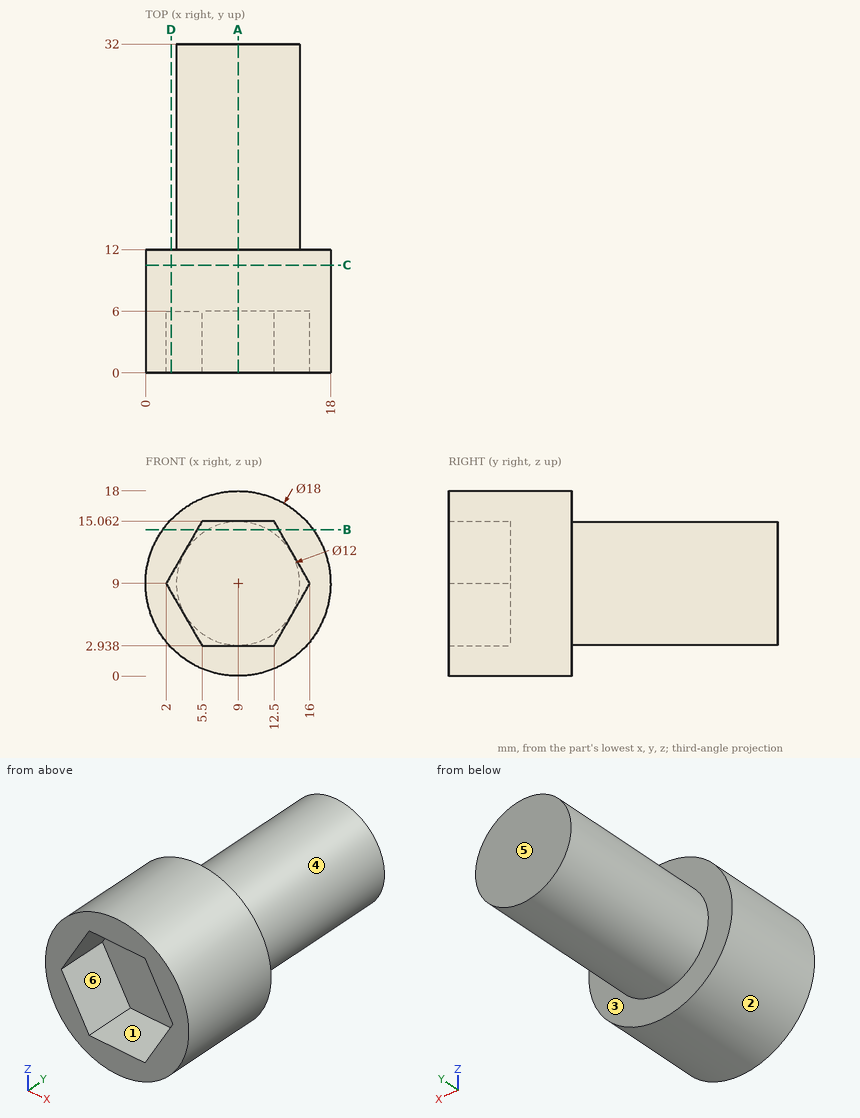
Job drawing, mm, ordinate dimensions from the low corner. One solid piece. A direction names the side the tool comes from. Round coordinates to 2 decimals unless told otherwise and drop trailing zeros. Write each loop counter-clockwise with the first axis right and the second up, starting at its lowest first coordinate (ties: lowest second). Pieces come first, ordered by that corner, then holes.
1) Band-saw the part on A-A, the plane x = 9. List the corners of the cut face in (y, z), and give its area (3 significant figures).
2) Band-saw the part on B-B, the plane z = 14.25. List the corners of the cut face in (x, y) (1 decimal).
3) Mould opens along Z. For the marked faces 4, 5 and 6 say: +Z half, -Z half, draft (parallel to the pull), parting line (faces both ways), or undercut.
4) Band-saw the part on D-D, the plane x = 2.5. List the corners of the cut face in (y, z) (3 decimals).
5) Band-saw the part on C-C, the plane y = 10.5. List the corners of the cut face in (x, z), and give its area (3 significant figures).
6) 3-axis set-ups, long thin cutter, end or side, ignore diameter. For the marked faces 1, 2 and 3: which of +Z, -Z, +X, -X, +Y, -Y reach the whole face in a straight line?
7) Pin check, flat tips, straight feed: pin 1 (10 mm diameter, centred on y = 27, z = 2.5, fed in from -X); pin 2 (1.8 mm diameter, centred on x = 10.5, y = 3, fed in from -Z); pin 3 (5 mm diameter, centred on y = 10.5, z = 3, fed in from +X). Stop position of each tip, or through.
8) Drill centre lines: probe 1 along Y at (x, z) = (14.25, 7.25); probe 2 along X at (y, z) = (12.5, 8.75) (1 decimal); probe 3 along Y at (x, z) = (4.5, 3.5). Where is each one in solid material? Low to high.
Ans:
1. outline: (0, 0) - (12, 0) - (12, 3) - (32, 3) - (32, 15) - (12, 15) - (12, 18) - (0, 18) - (0, 15.06) - (6, 15.06) - (6, 2.94) - (0, 2.94) - close
1. area: 383 mm2
2. outline: (1.7, 0) - (5, 0) - (5, 6) - (13, 6) - (13, 0) - (16.3, 0) - (16.3, 12) - (11.9, 12) - (11.9, 32) - (6.1, 32) - (6.1, 12) - (1.7, 12) - close
3. face 4: parting line
3. face 5: draft
3. face 6: undercut
4. outline: (0, 2.775) - (12, 2.775) - (12, 15.225) - (0, 15.225) - (0, 9.866) - (6, 9.866) - (6, 8.134) - (0, 8.134) - close
5. outline: circle Ø18 at (9, 9)
5. area: 254 mm2
6. face 1: -Y
6. face 2: +Y, -Y
6. face 3: +Y
7. pin 1: stops at x = 3.19
7. pin 2: stops at z = 0.02
7. pin 3: stops at x = 17.29
8. probe 1: y = 6 to 32
8. probe 2: x = 3 to 15
8. probe 3: y = 0 to 12
